from build123d import *

# Parameters (mm, degrees)
SKETCH1_W                = 25.4
SKETCH1_H                = 25.4
SKETCH1_W_2              = 23.4
SKETCH1_H_2              = 23.4
BOSS_EXTRUDE1_DEPTH      = 300
M6_CLEARANCE_HOLE1_D     = 6.6
M6_CLEARANCE_HOLE1_DEPTH = 10
M6_CLEARANCE_HOLE1_TIP   = 1.982840043
SKETCH5_W                = 12.861112754
SKETCH5_H                = 28
CUT_EXTRUDE2_DEPTH       = 10
M3_CLEARANCE_HOLE1_D     = 3.4
M3_CLEARANCE_HOLE1_DEPTH = 10
M3_CLEARANCE_HOLE1_TIP   = 1.021463052


with BuildPart() as part:
    # Sketch1 → Boss-Extrude1 (new body)
    with BuildSketch(Plane.XY):
        Rectangle(SKETCH1_W, SKETCH1_H)
        Rectangle(SKETCH1_W_2, SKETCH1_H_2, mode=Mode.SUBTRACT)
    extrude(amount=BOSS_EXTRUDE1_DEPTH)

    # M6 Clearance Hole1
    with Locations(Plane(origin=(0, 12.7, 0), x_dir=(1, 0, 0), z_dir=(0, 1, 0))):
        with Locations((0, -280), (0, -237.57)):
            Hole(M6_CLEARANCE_HOLE1_D / 2, depth=M6_CLEARANCE_HOLE1_DEPTH)
            with Locations((0, 0, -(M6_CLEARANCE_HOLE1_DEPTH + M6_CLEARANCE_HOLE1_TIP / 2))):  # 118° drill point
                Cone(0, M6_CLEARANCE_HOLE1_D / 2, M6_CLEARANCE_HOLE1_TIP, mode=Mode.SUBTRACT)

    # Sketch5 → Cut-Extrude2 (cut)
    with BuildSketch(Plane(origin=(0, 12.7, 0), x_dir=(1, 0, 0), z_dir=(0, 1, 0))):
        with Locations((0.3, -19)):
            Rectangle(SKETCH5_W, SKETCH5_H)
    extrude(amount=-CUT_EXTRUDE2_DEPTH, mode=Mode.SUBTRACT)

    # M3 Clearance Hole1
    with Locations(Plane(origin=(0, 12.7, 0), x_dir=(1, 0, 0), z_dir=(0, 1, 0))):
        with Locations((8.3, -2.320031624), (-7.7, -2.320031624), (-7.7, -35.340858472), (8.3, -35.340858472)):
            Hole(M3_CLEARANCE_HOLE1_D / 2, depth=M3_CLEARANCE_HOLE1_DEPTH)
            with Locations((0, 0, -(M3_CLEARANCE_HOLE1_DEPTH + M3_CLEARANCE_HOLE1_TIP / 2))):  # 118° drill point
                Cone(0, M3_CLEARANCE_HOLE1_D / 2, M3_CLEARANCE_HOLE1_TIP, mode=Mode.SUBTRACT)


solid = part.part
Work out the finished part from the listing and answer in its coordinate system (mm). A direction names the side the tool comes from. Round coordinates to 2 decimals unless told otherwise and drop trailing zeros. Write each loop counter-clockwise with the first axis right and the second up, starting at its lowest first coordinate (ties: lowest second). Pieces come first, ordered by that corner, then holes. Notation, with made-up numbers: (41.25, -17) -> (87.25, -17) arc R15 cw to (87.25, 12) -> close; hole circle Ø7 at (78, 69). An arc over 180 degrees is marked (long way). Answer as CSV lines item,"result". Start each with the question number.
(1) The part is cut by section B-B, the plane y = 9. Give the vertices of the cut face in (x, z), then the cut area to 3 significant figures.
(2) Find the intervals of material crossed by probe 1 along Z at (x, y) = (0, 12.55); probe 2 along X at (y, z) = (-4.25, 126), in increasing order.
(3) The part is cut by section D-D, the plane z = 280. Give the vertices of the cut face in (x, y), then the cut area to 3 significant figures.
(4) The part is cut by section C-C, the plane z = 71.5. Give the vertices of the cut face in (x, y).
(5) Each of these flat-tipped pins is pushed along its axis until it touches: pin 1 (6 mm diameter, centred on x = 0, z = 280, fed in from +Y); pin 2 (5 mm diameter, centred on x = -9, y = 3.5, fed in from -Z). Where does it stop, or does it pass through?
(6) The part is cut by section A-A, the plane x = 0. Give the vertices of the cut face in (y, z), then the cut area to 3 significant figures.
(7) The mould has two halves that part along Y. Classify faces 4 (the flat face through (0, 12.7, 148)), 5 (the flat face through (0, 11.7, 148)), 6 (the flat face through (-12.7, 0, 148)), 7 (the flat face through (0, -12.7, 148)): +Y half, -Y half, draft (parallel to the pull), parting line (faces both ways), or undercut.
(8) A tool of negligible diameter and unlimited length cuts with its end or side. For faces 1 (the cylindrical face through (-1.52, 12.19, 282.93)), 2 (the flat face through (-1, -12, 300)), 3 (the flat face through (11.7, 0, 148)), from which of +Z, -Z, +X, -X, +Y, -Y can it reach the whole face along a straight path? Write none if from no direction.
Output values:
1,outline,"(-12.7, 0) -> (-11.7, 0) -> (-11.7, 300) -> (-12.7, 300) -> close; (11.7, 0) -> (12.7, 0) -> (12.7, 300) -> (11.7, 300) -> close"
1,area,"600 mm²"
2,probe 1,"z = 0 to 5, 33 to 234.27, 240.87 to 276.7, 283.3 to 300"
2,probe 2,"x = -12.7 to -11.7, 11.7 to 12.7"
3,outline,"(-12.7, -12.7) -> (12.7, -12.7) -> (12.7, 12.7) -> (3.3, 12.7) -> (3.3, 11.7) -> (11.7, 11.7) -> (11.7, -11.7) -> (-11.7, -11.7) -> (-11.7, 11.7) -> (-3.3, 11.7) -> (-3.3, 12.7) -> (-12.7, 12.7) -> close"
3,area,"91.0 mm²"
4,outline,"(-12.7, -12.7) -> (12.7, -12.7) -> (12.7, 12.7) -> (-12.7, 12.7) -> close; hole (-11.7, -11.7) -> (11.7, -11.7) -> (11.7, 11.7) -> (-11.7, 11.7) -> close"
5,pin 1,"stops at y = -11.7"
5,pin 2,"passes through"
6,outline,"(-12.7, 0) -> (-11.7, 0) -> (-11.7, 300) -> (-12.7, 300) -> close; (11.7, 0) -> (12.7, 0) -> (12.7, 5) -> (11.7, 5) -> close; (11.7, 33) -> (12.7, 33) -> (12.7, 234.27) -> (11.7, 234.27) -> close; (11.7, 240.87) -> (12.7, 240.87) -> (12.7, 276.7) -> (11.7, 276.7) -> close; (11.7, 283.3) -> (12.7, 283.3) -> (12.7, 300) -> (11.7, 300) -> close"
6,area,"559 mm²"
7,face 4,"+Y half"
7,face 5,"undercut"
7,face 6,"draft"
7,face 7,"-Y half"
8,face 1,"+Y"
8,face 2,"+Z, +X, -X, +Y, -Y"
8,face 3,"+Z, -Z"
